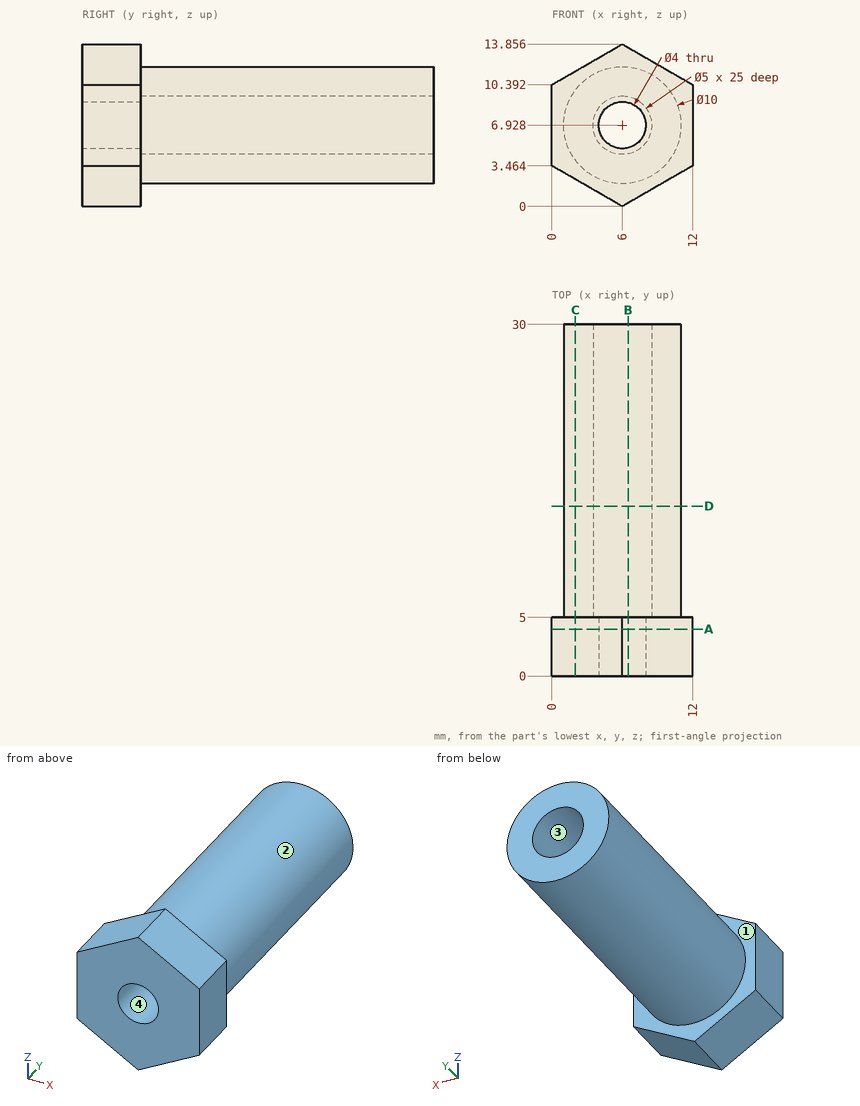
Study the drawing (mm; zero at the part's minimum x, y, z) and answer. Coordinates: 2 decimals unless noted, no trailing zeros. Order: outer loops, then holes, each group sorted by start corner. A loop starts at its lowest first (then second) coordinate and runs counter-clockwise, first axis right, second up. Notation, with made-up numbers: M 18.5,3.5 L 53.5,3.5 A31 cw 53.5,28.5 Z; hole C 56.5,61.25 d7. An arc over 180 degrees is marked long. Use CSV: the item, a comma, the result in double quotes.
Q1. Section C-C (x = 2) is taken. Determine the outline of the cut face in (y, z).
Here are the results:
outline,"M 0,2.31 L 5,2.31 L 5,3.93 L 30,3.93 L 30,9.93 L 5,9.93 L 5,11.55 L 0,11.55 Z"
Q2. Given pin 1 Ø2 at (x, y) = (7.5, 21.5) entering from -Z; pin 2 Ø2 at (y, z) = (10.5, 11.5) entering from +X; pin 3 Ø2 at (x, y) = (6, 21.5) entering from -Z, each flat-ended and moving along its own axis, determine where each tip first touches the part or whether it passes through.
Here are the results:
pin 1,"z = 1.95"
pin 2,"x = 9.5"
pin 3,"z = 1.93"
Q3. Section A-A (y = 4) is taken. Determine the outline of the cut face in (x, z).
Here are the results:
outline,"M 0,3.46 L 6,0 L 12,3.46 L 12,10.39 L 6,13.86 L 0,10.39 Z; hole C 6,6.93 d4"
Q4. Determine the mould class of the marked faces 1, 2, 3 and 4 for opening direction Z: pulls with the +Z half, pulls with the -Z half, needs draft (parallel to the pull), parting line crosses it, or undercut.
Here are the results:
face 1,"needs draft"
face 2,"parting line crosses it"
face 3,"undercut"
face 4,"undercut"
Q5. Section B-B (x = 6.5) is taken. Determine the outline of the cut face in (y, z) (1 decimal), then the cut area to 3 significant figures.
Here are the results:
outline,"M 0,0.3 L 5,0.3 L 5,2 L 30,2 L 30,4.5 L 5,4.5 L 5,5 L 0,5 Z; M 0,8.9 L 5,8.9 L 5,9.4 L 30,9.4 L 30,11.9 L 5,11.9 L 5,13.6 L 0,13.6 Z"
area,"173 mm2"
Q6. Section D-D (y = 14.5) is taken. Determine the outline of the cut face in (x, z), then the cut area to 3 significant figures.
Here are the results:
outline,"C 6,6.93 d10; hole C 6,6.93 d5"
area,"58.9 mm2"
Q7. Straight lines are drawn through the part: L1, parallel to X at y = 11.75, z = 5.25 (1 decimal); L2, parallel to X at y = 13, z = 5.75 (1 decimal); L3, parallel to Y at x = 5, z = 12.75. For each, find the intervals that lie inside material, in ascending order.
Here are the results:
L1,"1.3 to 4.1, 7.9 to 10.7"
L2,"1.1 to 3.8, 8.2 to 10.9"
L3,"0 to 5"
